```python
from build123d import *

# Parameters (mm, degrees)
F1_DEPTH  = 10
F3_DEPTH  = 13.6785106988
F4_DEPTH  = 3.268
F6_DEPTH  = 4
F8_DEPTH  = 4
F9_R      = 1.5
F10_DEPTH = 4.001


# Not quite as in the source:
# - a feature names something its author has since deleted; it is built from what else it names


with BuildPart() as f1:
    # F0 (on Top) → F1 (new body)
    with BuildSketch(Plane.XY):
        with BuildLine():
            Line((14.6115271971, -9.8928403326), (14.6115271971, -13.3118403326))
            Line((14.6115271971, -13.3118403326), (38.1115271971, -13.3118403326))
            Line((38.1115271971, -13.3118403326), (38.1115271971, -9.3118403326))
            Line((38.1115271971, -9.3118403326), (18.5955271971, -9.3118403326))
            ThreePointArc((18.5955271971, -9.3118403326), (8.3615271971, 0.3656703662), (-1.8724728029, -9.3118403326))
            Line((-1.8724728029, -9.3118403326), (-8.8884728029, -9.3118403326))
            Line((-8.8884728029, -9.3118403326), (-8.8884728029, -13.3118403326))
            Line((-8.8884728029, -13.3118403326), (2.1115271971, -13.3118403326))
            Line((2.1115271971, -13.3118403326), (2.1115271971, -9.8928403326))
            ThreePointArc((2.1115271971, -9.8928403326), (8.3615271971, -3.6428403326), (14.6115271971, -9.8928403326))
        make_face()
    extrude(amount=F1_DEPTH)

    # F2 (on face) → F3 (cut, through all)
    with BuildSketch(Plane.XZ.offset(13.3118403326)):
        Polygon((-2.1564728029, 5), (-3.0224728029, 6.4999559994), (-4.7544728029, 6.4999559994), (-5.6204728029, 5), (-4.7544728029, 3.5000440006), (-3.0224728029, 3.5000440006), align=None)
        Polygon((29.9775271971, 6.4999559994), (28.2455271971, 6.4999559994), (27.3795271971, 5), (28.2455271971, 3.5000440006), (29.9775271971, 3.5000440006), (30.8435271971, 5), align=None)
    extrude(amount=-F3_DEPTH, mode=Mode.SUBTRACT)

    # F4 (cut): a face of the model
    f4_faces = [f1.faces().sort_by_distance(p)[0] for p in [
        (38.1115271971, -11.3118403326, 5),
    ]]
    extrude(f4_faces, amount=-F4_DEPTH, mode=Mode.SUBTRACT)

    # F5 (on face) → F6 (join, through all)
    with BuildSketch(Plane(origin=(0, -9.3118403326, 0), x_dir=(-1, 0, 0), z_dir=(0, 1, 0))):
        Polygon((4.7544728029, 3.5000440006), (5.6204728029, 5), (4.7544728029, 6.4999559994), (3.0224728029, 6.4999559994), (2.1564728029, 5), (3.0224728029, 3.5000440006), align=None)
    extrude(amount=-F6_DEPTH)

    # F7 (on face) → F8 (join, through all)
    with BuildSketch(Plane(origin=(0, -9.3118403326, 0), x_dir=(-1, 0, 0), z_dir=(0, 1, 0))):
        Polygon((-28.2455271971, 3.5000440006), (-27.3795271971, 5), (-28.2455271971, 6.4999559994), (-29.9775271971, 6.4999559994), (-30.8435271971, 5), (-29.9775271971, 3.5000440006), align=None)
    extrude(amount=-F8_DEPTH)

    # F9 (on face) → F10 (cut, through all)
    with BuildSketch(Plane(origin=(0, -9.3118403326, 0), x_dir=(-1, 0, 0), z_dir=(0, 1, 0))):
        with Locations((5.3804728029, 5)):
            Circle(F9_R)
        with Locations((-26.7195271971, 5)):
            Circle(F9_R)
    extrude(amount=-F10_DEPTH, mode=Mode.SUBTRACT)


solid = f1.part
```
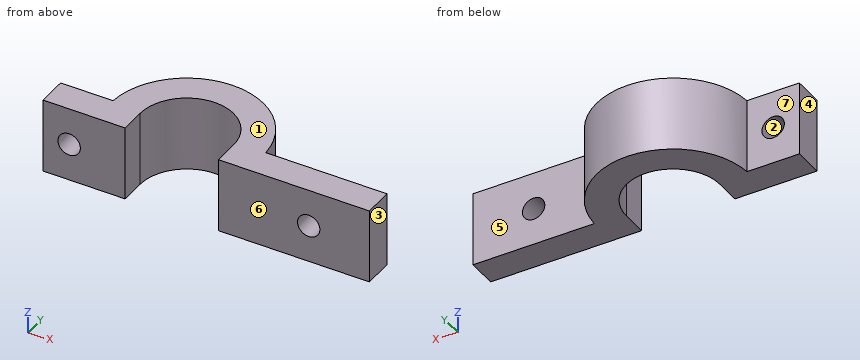
The listing builds one solid part. Answer for the finished solid, in the listing's coordinates (mm). Face numbers are marked on the shaded views. A direction names the side the tool comes from. Coordinates: 2 decimals unless noted, no trailing zeros. Loops run counter-clockwise (first coordinate to the right, second up) from the corner with the lowest first, then second, coordinate; pieces in that order, holes last. Notation, with made-up numbers: (42.5, -22) -> (98.5, -22) arc R31 cw to (98.5, 10) -> close; hole circle Ø6 at (85.25, -36). An arc over 180 degrees is marked (long way). Return JSON: item names as keys, results as strings. Group by question number.
(1) A cutting plane is placed at A-A on y = -11.75. Write down the section's boundary in (x, z), and give its area (3 significant figures).
(2) Determine the mould class of the marked faces 1, 2, 3 and 4 for opening direction X: released by +X, released by -X, zero draft, split by the parting line, or undercut.
(3) Find the intervals of material crossed by probe 1 along X at (y, z) = (-10.25, 0.5); probe 2 along Y at (x, z) = (28.5, 1.5); probe 3 along X at (y, z) = (-4.5, 8), in increasing order. Write a range as from..to.
(4) Which of the six approach directions +Z, -Z, +X, -X, +Y, -Y give full straight-line access (tool end or side, diameter ignored) to the marked faces 5, 6 and 7?
(5) A cutting plane is placed at B-B on z = 5. Write down the section's boundary in (x, y), and give its area (3 significant figures).
(6) A cutting plane is placed at C-C on y = -4.5. Write down the section's boundary in (x, z).
(7) Given pin 1 Ø2 at (x, z) = (-1.5, 8) entering from +Y; pin 2 Ø5 at (x, y) = (-3.5, -8.5) entering from +Z; pin 3 Ø2.5 at (x, z) = (-5.38, 5) entering from +Y; pin 4 Ø4 at (x, z) = (26.72, 5) entering from +Y, each flat-ended and moving along its own axis, determine where each tip first touches the part or whether it passes through.
(8) A cutting plane is placed at D-D on z = 2. Write down the section's boundary in (x, y).
The answers:
{
 "1": {"outline": "(-8.89, 0) -> (2.11, 0) -> (2.11, 10) -> (-8.89, 10) -> close; (14.61, 0) -> (34.84, 0) -> (34.84, 10) -> (14.61, 10) -> close; hole circle Ø3 at (-5.38, 5); hole circle Ø3 at (26.72, 5)", "area": "298 mm^2"},
 "2": {"face 1": "zero draft", "face 2": "undercut", "face 3": "released by +X", "face 4": "released by -X"},
 "3": {"probe 1": "x = -8.89..2.11, 14.61..34.84", "probe 2": "y = -13.31..-9.31", "probe 3": "x = -0.36..5.2, 11.52..17.08"},
 "4": {"face 5": "+Z, -Z, +X, +Y", "face 6": "+Z, -Z, +X, -X, -Y", "face 7": "+Z, -Z, -X, +Y"},
 "5": {"outline": "(-8.89, -13.31) -> (-6.88, -13.31) -> (-6.88, -9.31) -> (-8.89, -9.31) -> close; (-3.88, -13.31) -> (2.11, -13.31) -> (2.11, -9.89) arc R6.25 cw to (14.61, -9.89) -> (14.61, -13.31) -> (25.22, -13.31) -> (25.22, -9.31) -> (18.6, -9.31) arc R10.25 ccw to (-1.87, -9.31) -> (-3.88, -9.31) -> close; (28.22, -13.31) -> (34.84, -13.31) -> (34.84, -9.31) -> (28.22, -9.31) -> close", "area": "200 mm^2"},
 "6": {"outline": "(-0.36, 0) -> (5.2, 0) -> (5.2, 10) -> (-0.36, 10) -> close; (11.52, 0) -> (17.08, 0) -> (17.08, 10) -> (11.52, 10) -> close"},
 "7": {"pin 1": "stops at y = -4.73", "pin 2": "stops at z = 10", "pin 3": "passes through", "pin 4": "stops at y = -9.31"},
 "8": {"outline": "(-8.89, -13.31) -> (2.11, -13.31) -> (2.11, -9.89) arc R6.25 cw to (14.61, -9.89) -> (14.61, -13.31) -> (34.84, -13.31) -> (34.84, -9.31) -> (18.6, -9.31) arc R10.25 ccw to (-1.87, -9.31) -> (-8.89, -9.31) -> close"}
}
